Check sheet for the drawn part. Datum: minimum x, y, z corner. Units: mm. A direction names the side the tool comes from. Coordinates: 2 decimals unless noted, no trailing zeros. Loops run counter-clockwise (first coordinate to the right, second up) from the corner with the lowest first, then second, coordinate; pieces in that order, holes last.
Q1. Go/stop test with flat-tipped pins: P1, Ø5, axis at y = 17.5, z = 218.5, coming from the -X side; P2, Ø4, axis at y = 28.5, z = 143.5, coming from the +X side; P3, Ø1, axis at x = 259, z = 79, coming from the -Y side. Record where each tip stops, or that it passes through.
Q2. Sectioned sample at B-B (y = 31). Enter the section's corners in (x, z).
Q3. Sectioned sample at A-A (z = 57.5). Enter the section's corners in (x, y) (3 decimals), then the cut area to 3 significant figures.
Q4. Material ranges on probe 1 along X at (y, z) = (19.05, 85.5) (3 decimals); probe 2 along Y at (x, z) = (82.55, 132) (3 decimals); probe 3 along Y at (x, z) = (125, 244), recorded low to high.
Q5. Access from +Z, -Z, +X, -X, +Y, -Y to the whole of each face (thin tool, end or side, straight path). Record for the marked faces 1, 2 and 3.
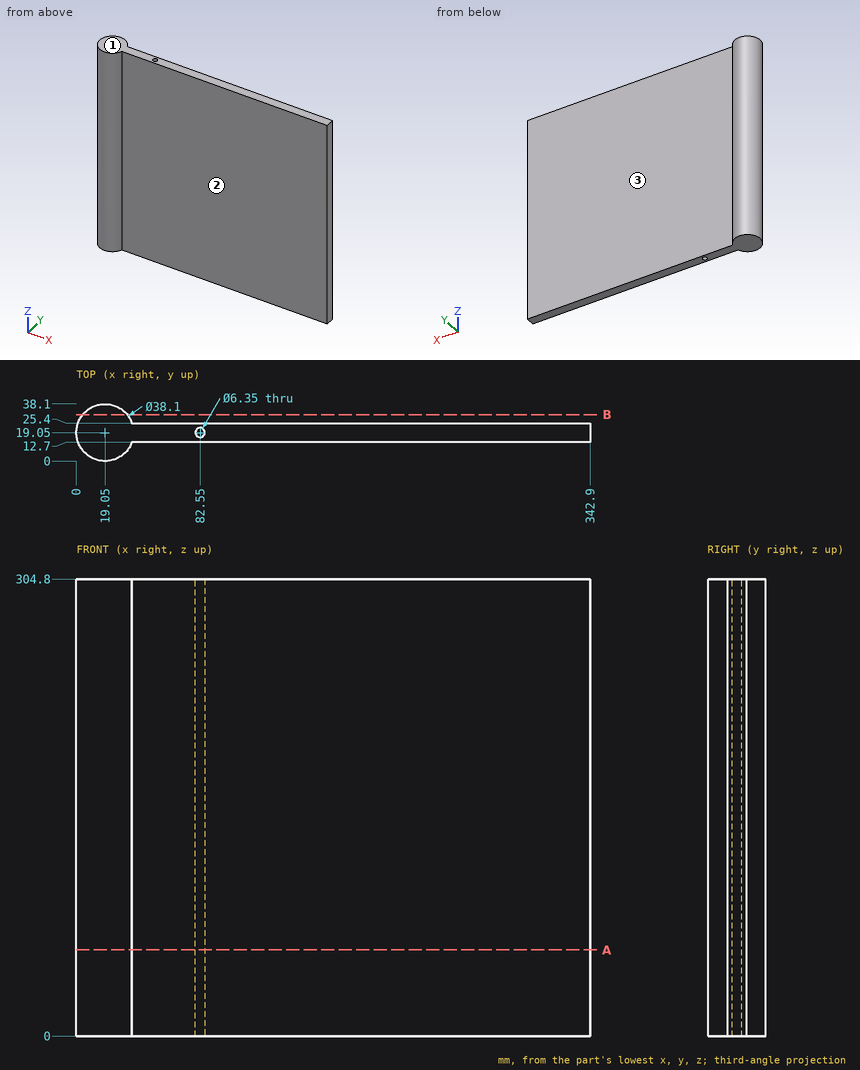
Geometry check:
1. P1: stops at x = 0
1. P2: stops at x = 36.58
1. P3: stops at y = 12.7
2. outline: (4.21, 0) - (33.89, 0) - (33.89, 304.8) - (4.21, 304.8) - close
3. outline: (37.011, 12.7) - (342.9, 12.7) - (342.9, 25.4) - (37.011, 25.4) arc R19.05 ccw (long way) to start; hole circle Ø6.35 at (82.55, 19.05)
3. area: 4,980 mm2
4. probe 1: x = 0 to 79.375, 85.725 to 342.9
4. probe 2: y = 12.7 to 15.875, 22.225 to 25.4
4. probe 3: y = 12.7 to 25.4
5. face 1: +Z, +X, -X, +Y, -Y
5. face 2: +Z, -Z, +X, -Y
5. face 3: +Z, -Z, +X, +Y
